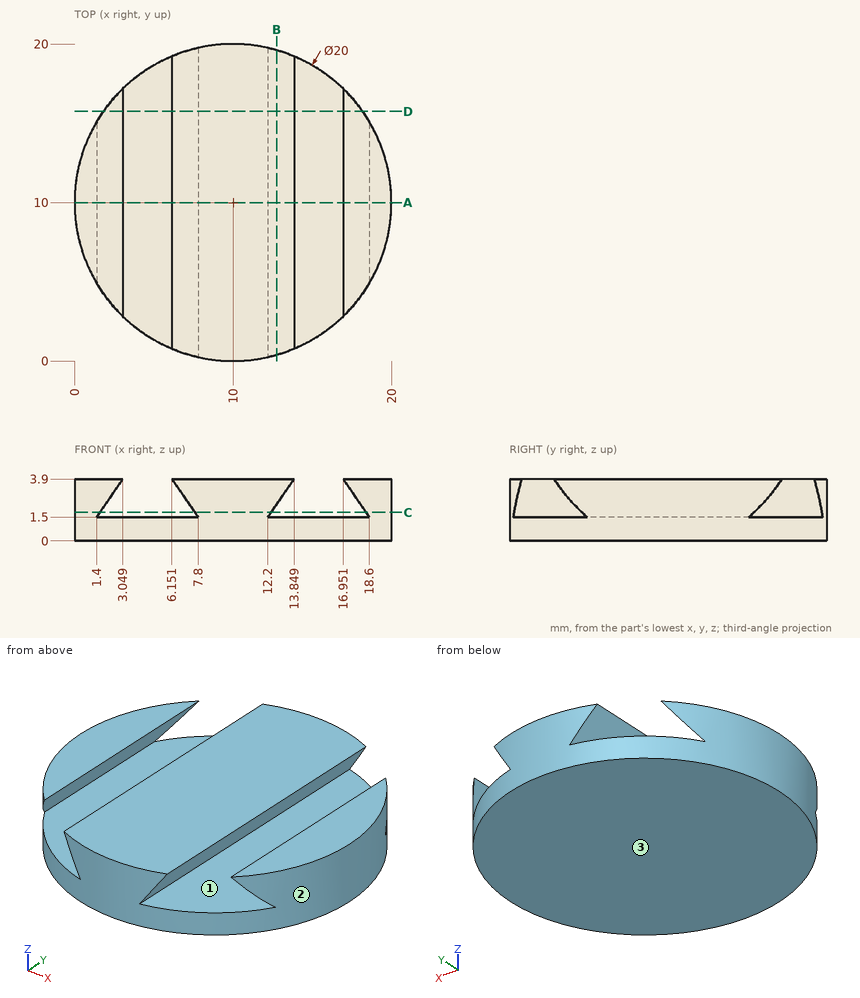
Print and shaded views of the part. All mm, measured from the part's lowest x, y and z. Coordinates: 2 decimals unless noted, no trailing zeros. Loops run counter-clockwise (first coordinate to the right, second up) from the corner with the lowest first, then second, coordinate; pieces in that order, holes last. Notation, with made-up numbers: (13.25, 58.5) -> (61.25, 58.5) arc R29 ccw to (61.25, 79.5) -> close; hole circle Ø8 at (87.5, 31). An arc over 180 degrees is marked (long way). Use one line per item in the form item = value. Start each with the question number.
(1) Flat gauge pins, fed straight in: pin 1 (1 mm diameter, centred on y = 16, z = 3.5, fed in from +X); pin 2 (1 mm diameter, centred on x = 8, z = 1.5, fed in from +Y). Where does each tip first touch, or does it go through?
(2) Cut at A-A on y = 10. Give the cut face in (x, z).
(3) Cut at C-C on z = 1.8. Give the cut face in (x, y) (1 decimal), and give its area (3 significant figures).
(4) Pull direction X, two halves, no side cores. Call the marked faces 1, 2 and 3: pulls with the +X half, pulls with the -X half, needs draft (parallel to the pull), parting line crosses it, or undercut.
(5) Cut at B-B on x = 12.75. Give the cut face in (y, z) (1 decimal).
(6) Cut at D-D on y = 15.75. Give the cut face in (x, z).
(7) Probe probe 1 along X at (y, z) = (5.5, 1.75); probe 2 along Z at (x, y) = (5.5, 9); probe 3 along Z at (x, y) = (7, 15) (1 decimal). List the from-to ranges inside material, lowest first. Write a range as from..to.
Values:
q1.pin_1 = 18.35
q1.pin_2 = 19.89
q2.outline = (0, 0) -> (20, 0) -> (20, 3.9) -> (16.95, 3.9) -> (18.6, 1.5) -> (12.2, 1.5) -> (13.85, 3.9) -> (6.15, 3.9) -> (7.8, 1.5) -> (1.4, 1.5) -> (3.05, 3.9) -> (0, 3.9) -> close
q3.outline = (1.6, 4.6) -> (1.6, 15.4) arc R10 ccw to start; (7.6, 0.3) arc R10 ccw to (12.4, 0.3) -> (12.4, 19.7) arc R10 ccw to (7.6, 19.7) -> close; (18.4, 4.6) arc R10 ccw to (18.4, 15.4) -> close
q3.area = 119 mm2
q4.face_1 = undercut
q4.face_2 = parting line crosses it
q4.face_3 = needs draft
q5.outline = (0.4, 0) -> (19.6, 0) -> (19.6, 1.5) -> (0.4, 1.5) -> close; (0.4, 2.3) -> (19.6, 2.3) -> (19.6, 3.9) -> (0.4, 3.9) -> close
q6.outline = (1.82, 0) -> (18.18, 0) -> (18.18, 1.5) -> (12.2, 1.5) -> (13.85, 3.9) -> (6.15, 3.9) -> (7.8, 1.5) -> (1.82, 1.5) -> close; (1.82, 2.11) -> (3.05, 3.9) -> (1.82, 3.9) -> close; (16.95, 3.9) -> (18.18, 2.11) -> (18.18, 3.9) -> close
q7.probe_1 = 1.07..1.57, 7.63..12.37, 18.43..18.93
q7.probe_2 = 0..1.5
q7.probe_3 = 0..1.5, 2.7..3.9
